Work out the finished part from the listing and answer in its coordinate system (mm). Round coordinates to 2 decimals unless told otherwise and drop trailing zeros. Loops run counter-clockwise (first coordinate to the right, second up) from the corner with the lowest first, then second, coordinate; pieces in that order, holes last. Notation, with made-up numbers: (16, 22) - (61, 22) arc R17 ccw to (61, 44) - close; hole circle Ø10 at (-2.5, -2.75). An arc over 180 degrees is marked (long way). Return JSON: item names as keys, results as strings.
from build123d import *

# Parameters (mm, degrees)
F0_R     = 25.4
F0_R_2   = 19.05
F1_DEPTH = 508
F4_R     = 6.35
F5_DEPTH = 25.4
F3_R     = 6.35
F6_DEPTH = 25.4


with BuildPart() as f1:
    # F0 (on Front) → F1 (new body, symmetric)
    with BuildSketch(Plane.XZ):
        Circle(F0_R)
        Circle(F0_R_2, mode=Mode.SUBTRACT)
    extrude(amount=F1_DEPTH, both=True)

    # F4 (on Top) → F5 (cut)
    with BuildSketch(Plane.XY):
        with Locations((0, 488.95)):
            Circle(F4_R)
        with Locations((0, 266.7)):
            Circle(F4_R)
    extrude(amount=-F5_DEPTH, mode=Mode.SUBTRACT)

    # F3 (on Right) → F6 (cut, symmetric)
    with BuildSketch(Plane.YZ):
        with Locations((381, 0)):
            Circle(F3_R)
    extrude(amount=F6_DEPTH, both=True, mode=Mode.SUBTRACT)


solid = f1.part
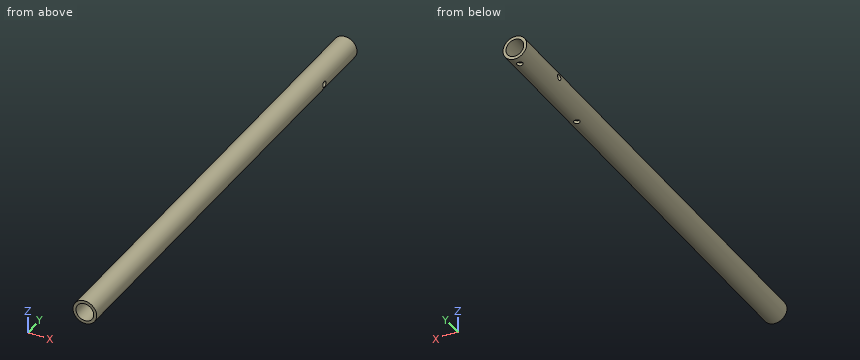
1) Find the intervals of material crossed by L1, parallel to Y at x = 0, z = -20.5; L2, parallel to Z at x = -1, y = -317; L3, parallel to X at y = -302, z = 0, in increasing order.
Verdict:
{"L1": "y = -508 to 260.35, 273.05 to 482.6, 495.3 to 508", "L2": "z = -25.38 to -19.02, 19.02 to 25.38", "L3": "x = -25.4 to -19.05, 19.05 to 25.4"}
2) Flat-ended cylindrical pins translate along their axes: pin 1 (5 mm diameter, centred on x = 5, y = -187.5, fed in from +Z); pin 2 (8 mm diameter, centred on y = -128, z = -10, fed in from -X); pin 3 (1.5 mm diameter, centred on x = -2, y = -331.5, fed in from -Z). Find the tip coordinate at first contact, or state that the pin passes through.
Verdict:
{"pin 1": "stops at z = 25.28", "pin 2": "stops at x = -24.68", "pin 3": "stops at z = -25.37"}
3) Section A-A (y = -304.5) is taken. Give the vertices of the cut face in (x, z).
Verdict:
{"outline": "circle Ø50.8 at (0, 0); hole circle Ø38.1 at (0, 0)"}
